Geometry check sheet. Reference: the model listing, model coordinates, mm. A direction names the side the tool comes from. Give positions to 0.01 mm unless a question says otherwise; leave off trailing zeros. Loops run counter-clockwise (first coordinate to the right, second up) from the corner with the lowest first, then second, coordinate; pieces in that order, holes last.
1. Cross-section at A-A, the plane x = -81.28. Record the cut outline in (y, z) (3 decimals), plus the area to 3 significant figures.
2. Tool access check on faces 1 (the cylindrical face through (-31.918, 0.287, 25.044)), 2 (the cylindrical face through (-70.972, -12.177, 44.539)). Record the directions out of +Z, -Z, +X, -X, +Y, -Y that give a thin tool (end or side, any length) a straight path to the whole face; none if there is none.
3. Cross-section at B-B, the plane z = 28. Record the cut outline in (x, y) (3 decimals).
4. Material ranges on L1, parallel to Y at x = -25.4, z = 17 (3 decimals); L2, parallel to Y at x = -81, z = 38 (3 decimals); L3, parallel to X at y = -30.5, z = 38.5, recorded low to high.
5. Go/stop test with a flat-tipped pin: pin 1 Ø22 at (x, y) = (-56.5, -25) entering from +Z. Record where the tip stops, or that it passes through.
6. Cross-section at D-D, the plane z = 44.5. Record the cut outline in (x, y) (3 decimals), plus the area to 3 significant figures.
7. Release check for a two-part mould opening along X. For faces 3 (the cylindrical face through (76.473, 4.408, 25.044)), 4 (the flat face through (101.6, -4, 25)), 5 (the flat face through (-1, -2, 50.8)), 6 (the flat face through (-101.6, -3, 25)) record: +X half, -X half, draft (parallel to the pull), parting line (faces both ways), or undercut.
8. Cross-section at C-C, the plane x = 81.28. Record the cut outline in (y, z) (3 decimals), plus the area to 3 significant figures.
from build123d import *

# Parameters (mm, degrees)
F0_R     = 5.787016
F0_R_2   = 6.524432
F0_R_3   = 6.27749
F0_R_4   = 6.521669
F1_DEPTH = 50.8
F2_R     = 22.123373
F2_R_2   = 17.63113
F3_DEPTH = 12.7


with BuildPart() as f1:
    # F0 (on Top) → F1 (new body)
    with BuildSketch(Plane.XY):
        with BuildLine():
            ThreePointArc((-101.6, -50.8), (-100.670064, -53.045064), (-98.425, -53.975))
            Line((-98.425, -53.975), (98.425, -53.975))
            ThreePointArc((98.425, -53.975), (100.670064, -53.045064), (101.6, -50.8))
            Line((101.6, -50.8), (101.6, 44.45))
            ThreePointArc((101.6, 44.45), (100.670064, 46.695064), (98.425, 47.625))
            Line((98.425, 47.625), (-98.425, 47.625))
            ThreePointArc((-98.425, 47.625), (-100.670064, 46.695064), (-101.6, 44.45))
            Line((-101.6, 44.45), (-101.6, -50.8))
        make_face()
        with Locations((-81.28, 0)):
            Circle(F0_R, mode=Mode.SUBTRACT)
        with Locations((-25.4, 0)):
            Circle(F0_R_2, mode=Mode.SUBTRACT)
        with Locations((25.4, 0)):
            Circle(F0_R_3, mode=Mode.SUBTRACT)
        with Locations((81.28, 0)):
            Circle(F0_R_4, mode=Mode.SUBTRACT)
    extrude(amount=F1_DEPTH)

    # F2 (on face) → F3 (cut)
    with BuildSketch(Plane.XY.offset(50.8)):
        with Locations((-54.665826, -27.128531)):
            Circle(F2_R)
        with Locations((47.767427, -21.433132)):
            Circle(F2_R_2)
    extrude(amount=-F3_DEPTH, mode=Mode.SUBTRACT)


solid = f1.part
Result:
1. outline: (-53.975, 0) - (-5.787, 0) - (-5.787, 50.8) - (-53.975, 50.8) - close; (5.787, 0) - (47.625, 0) - (47.625, 50.8) - (5.787, 50.8) - close
1. area: 4,570 mm2
2. face 1: +Z, -Z
2. face 2: +Z
3. outline: (-101.6, -50.8) arc R3.175 ccw to (-98.425, -53.975) - (98.425, -53.975) arc R3.175 ccw to (101.6, -50.8) - (101.6, 44.45) arc R3.175 ccw to (98.425, 47.625) - (-98.425, 47.625) arc R3.175 ccw to (-101.6, 44.45) - close; hole circle Ø11.574 at (-81.28, 0); hole circle Ø13.049 at (-25.4, 0); hole circle Ø12.555 at (25.4, 0); hole circle Ø13.043 at (81.28, 0)
4. L1: y = -53.975 to -6.524, 6.524 to 47.625
4. L2: y = -53.975 to -5.78, 5.78 to 47.625
4. L3: x = -101.6 to -76.53, -32.8 to 32.65, 62.89 to 101.6
5. pin 1: stops at z = 38.1
6. outline: (-101.6, -50.8) arc R3.175 ccw to (-98.425, -53.975) - (98.425, -53.975) arc R3.175 ccw to (101.6, -50.8) - (101.6, 44.45) arc R3.175 ccw to (98.425, 47.625) - (-98.425, 47.625) arc R3.175 ccw to (-101.6, 44.45) - close; hole circle Ø11.574 at (-81.28, 0); hole circle Ø44.247 at (-54.666, -27.129); hole circle Ø13.049 at (-25.4, 0); hole circle Ø12.555 at (25.4, 0); hole circle Ø35.262 at (47.767, -21.433); hole circle Ø13.043 at (81.28, 0)
6. area: 17,600 mm2
7. face 3: undercut
7. face 4: +X half
7. face 5: draft
7. face 6: -X half
8. outline: (-53.975, 0) - (-6.522, 0) - (-6.522, 50.8) - (-53.975, 50.8) - close; (6.522, 0) - (47.625, 0) - (47.625, 50.8) - (6.522, 50.8) - close
8. area: 4,500 mm2
